The listing builds one solid part. Answer for the finished solid, in the listing's coordinates (mm). Face numbers are marked on the shaded views. A direction names the side the tool comes from. Coordinates: 2 decimals unless noted, no trailing zeros. Order: outer loops, then holes, each group sorted by start corner. A loop starts at its lowest first (then second) coordinate and runs counter-clockwise, first axis right, second up. Notation, with made-up numbers: (77.5, -3) -> (127.5, -3) arc R32 cw to (127.5, 26) -> close; hole circle Ø11 at (65, 20.5). An arc over 180 degrees is marked (long way). Write item = value, one per line.
Autodesk Inventor part; units mm, degrees
ref_plane "YZ Plane" through (0, 0, 0) normal (1, 0, 0) x (0, 1, 0)
ref_plane "XZ Plane" through (0, 0, 0) normal (0, 1, 0) x (-1, 0, 0)
ref_plane "XY Plane" through (0, 0, 0) normal (0, 0, 1) x (1, 0, 0)
sketch "草圖1" plane through (0, 0, 0) normal (0, 1, 0) x (-1, 0, 0)
  circle A0 centre (0, 0) radius 14
  circle A1 centre (0, 0) radius 10
  circle A2 centre (10, 0) radius 1.75
  circle A3 centre (0, 10) radius 1.75
  circle A4 centre (-10, 0) radius 1.75
  circle A5 centre (0, -10) radius 1.75
  dimension "d3" = 20
  dimension "d0" = 28
  dimension "d4" = 3.5
  dimension "d7" = 360
extrude "擠出1" add sketch "草圖1" along normal blind 5 contours A0 | A2 A1 A5 A4 A3
sketch "草圖2" plane through (0, 5, 0) normal (0, 1, 0) x (1, 0, 0)
  circle A0 centre (0, 0) radius 6
  dimension "d9" = 12
extrude "擠出2" add sketch "草圖2" along normal blind 11
sketch "草圖3" plane through (0, 16, 0) normal (0, 1, 0) x (1, 0, 0)
  circle A0 centre (0, 0) radius 4
  dimension "d12" = 8
extrude "擠出3" cut sketch "草圖3" against normal through all
properties part number "8mm axle mount"
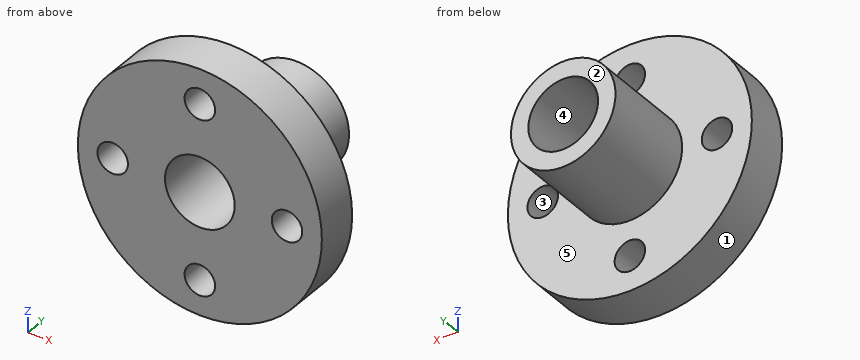
Q1. The mould has two halves that part along X. Classify the marked faces 1, 2 and 3: released by +X, released by -X, zero draft, split by the parting line, or undercut.
The answers:
face_1 = split by the parting line
face_2 = zero draft
face_3 = undercut
Q2. Section B-B, the plane x = 0 is taken. Give the vertices of the cut face in (y, z), plus the area to 3 significant figures.
The answers:
outline = (0, -14) -> (5, -14) -> (5, -11.75) -> (0, -11.75) -> close; (0, -8.25) -> (5, -8.25) -> (5, -6) -> (16, -6) -> (16, -4) -> (0, -4) -> close; (0, 4) -> (16, 4) -> (16, 6) -> (5, 6) -> (5, 8.25) -> (0, 8.25) -> close; (0, 11.75) -> (5, 11.75) -> (5, 14) -> (0, 14) -> close
area = 109 mm2
Q3. A tool of negligible diameter and unlimited length cuts with its end or side. For the marked faces 4 and 5, from which of +Z, -Z, +X, -X, +Y, -Y can it reach the whole face along a straight path? Write none if from no direction.
The answers:
face_4 = +Y, -Y
face_5 = +Y
Q4. Section C-C, the plane z = 9 is taken. Give the vertices of the cut face in (x, y).
The answers:
outline = (-10.72, 0) -> (-1.44, 0) -> (-1.44, 5) -> (-10.72, 5) -> close; (1.44, 0) -> (10.72, 0) -> (10.72, 5) -> (1.44, 5) -> close
Q5. Each of these flat-tipped pins is pushed along its axis until it touches: pin 1 Ø4.5 at (x, z) = (0, 10) entering from +Y; pin 2 Ø3 at (x, z) = (-10, 0) entering from -Y; pin 3 Ø1.5 at (x, y) = (-5, 9) entering from +Z; pin 4 Ø6 at (x, y) = (-6.5, 12.5) entering from +Z. Where does it stop, or does it pass through?
The answers:
pin_1 = 5
pin_2 = through
pin_3 = 4.24
pin_4 = 4.87
Q6. Section A-A, the plane z = 0 is taken. Give the vertices of the cut face in (x, y).
The answers:
outline = (-14, 0) -> (-11.75, 0) -> (-11.75, 5) -> (-14, 5) -> close; (-8.25, 0) -> (-4, 0) -> (-4, 16) -> (-6, 16) -> (-6, 5) -> (-8.25, 5) -> close; (4, 0) -> (8.25, 0) -> (8.25, 5) -> (6, 5) -> (6, 16) -> (4, 16) -> close; (11.75, 0) -> (14, 0) -> (14, 5) -> (11.75, 5) -> close
Q7. Find the intervals of material crossed by line 1 along Z through (x, y) = (0, 2.55); line 2 along Z through (x, y) = (0, 10.25); line 3 along Y through (x, z) = (-1.5, -6), in increasing order.
The answers:
line_1 = -14 to -11.75, -8.25 to -4, 4 to 8.25, 11.75 to 14
line_2 = -6 to -4, 4 to 6
line_3 = 0 to 5
Q8. Section D-D, the plane y = 1.5 is taken. Give the vertices of the cut face in (x, z).
The answers:
outline = circle Ø28 at (0, 0); hole circle Ø3.5 at (-10, 0); hole circle Ø8 at (0, 0); hole circle Ø3.5 at (0, -10); hole circle Ø3.5 at (0, 10); hole circle Ø3.5 at (10, 0)
